Verification items for the finished model (mm, model axes). A direction names the side the tool comes from. Coordinates: 2 decimals unless noted, no trailing zeros. Order: outer loops, then holes, each group sorted by start corner. A loop starts at its lowest first (then second) coordinate and runs counter-clockwise, first axis right, second up. Notation, with made-up numbers: M 4.25,88.25 L 52.25,88.25 A21 ccw 52.25,120.25 Z; hole C -37,34 d9. An arc over 180 degrees is marked long. Use one line per item in the form item = value. Start each with the question number.
```python
from build123d import *

# Parameters (mm, degrees)
BOSS_EXTRUDE1_DEPTH      = 32.1
SKETCH2_R                = 3.075
BOSS_EXTRUDE2_DEPTH      = 1.6
BOSS_EXTRUDE3_START      = 2.1
SKETCH3_R                = 3.075
BOSS_EXTRUDE3_DEPTH      = 2.1
M2_TAPPED_HOLE1_D        = 1.6
M2_TAPPED_HOLE1_DEPTH    = 6
M2_TAPPED_HOLE1_TIP      = 0.480688495
SKETCH6_R                = 1.2
SKETCH6_R_2              = 1.5
BOSS_EXTRUDE4_DEPTH      = 1
SKETCH7_R                = 1
BOSS_EXTRUDE5_DEPTH      = 6
FILLET1_R                = 1
FILLET2_R                = 0.5
BOSS_EXTRUDE6_DEPTH      = 0.15
BOSS_EXTRUDE6_DEPTH_BACK = 0.15
SKETCH9_W                = 1.4
SKETCH9_H                = 1.4
FILLET3_R                = 0.5


with BuildPart() as part:
    # Sketch1 → Boss-Extrude1 (new body)
    with BuildSketch(Plane.XY):
        with BuildLine():
            Line((-6.68954408, 7.7), (6.68954408, 7.7))
            ThreePointArc((6.68954408, 7.7), (10.2, 0), (6.68954408, -7.7))
            Line((6.68954408, -7.7), (-6.68954408, -7.7))
            ThreePointArc((-6.68954408, -7.7), (-10.2, 0), (-6.68954408, 7.7))
        make_face()
    extrude(amount=BOSS_EXTRUDE1_DEPTH)

    # Sketch2 → Boss-Extrude2 (add)
    with BuildSketch(Plane.XY.offset(32.1)):
        Circle(SKETCH2_R)
    extrude(amount=BOSS_EXTRUDE2_DEPTH)

    # Sketch3 → Boss-Extrude3 (add)
    with BuildSketch(Plane(origin=(0, 0, 0), x_dir=(-1, 0, 0), z_dir=(0, 0, -1)).offset(BOSS_EXTRUDE3_START)):
        with Locations(Location((0, 0, 0), (0, 0, 180))):
            Circle(SKETCH3_R)
    extrude(amount=-BOSS_EXTRUDE3_DEPTH)

    # M2 Tapped Hole1
    with Locations(Plane.XY.offset(32.1)):
        with Locations((-6.2, 0), (6.2, 0)):
            Hole(M2_TAPPED_HOLE1_D / 2, depth=M2_TAPPED_HOLE1_DEPTH)
            with Locations((0, 0, -(M2_TAPPED_HOLE1_DEPTH + M2_TAPPED_HOLE1_TIP / 2))):  # 118° drill point
                Cone(0, M2_TAPPED_HOLE1_D / 2, M2_TAPPED_HOLE1_TIP, mode=Mode.SUBTRACT)

    # Sketch6 → Boss-Extrude4 (add)
    with BuildSketch(Plane(origin=(0, 0, 0), x_dir=(-1, 0, 0), z_dir=(0, 0, -1))):
        with Locations(Location((-7.6, 1.69, 0), (0, 0, 180))):
            Circle(SKETCH6_R)
        with Locations(Location((7.6, -1.69, 0), (0, 0, 180))):
            Circle(SKETCH6_R)
        with Locations(Location((-7.6, -1.69, 0), (0, 0, 180))):
            Circle(SKETCH6_R_2)
        with Locations(Location((7.6, 1.69, 0), (0, 0, 180))):
            Circle(SKETCH6_R_2)
    extrude(amount=BOSS_EXTRUDE4_DEPTH)

    # Sketch7 → Boss-Extrude5 (add)
    with BuildSketch(Plane.XY.offset(33.7)):
        Circle(SKETCH7_R)
    extrude(amount=BOSS_EXTRUDE5_DEPTH)

    # Fillet1
    fillet1_edges = [part.edges().sort_by_distance(p)[0] for p in [
        (-10.2, 0, 32.1),
        (0, -7.7, 32.1),
        (10.2, 0, 32.1),
        (0, 7.7, 32.1),
    ]]
    fillet(fillet1_edges, radius=FILLET1_R)

    # Fillet2
    fillet2_edges = [part.edges().sort_by_distance(p)[0] for p in [
        (-3.075, 0, 0),
        (-3.075, 0, -2.1),
    ]]
    fillet(fillet2_edges, radius=FILLET2_R)

    # Sketch9 → Boss-Extrude6 (add, two sides: drawn at the far end of the back side and taken through both)
    # profile 1 of 2: a face of its own
    with BuildSketch(Plane(origin=(0, 0, 0), x_dir=(-0.9761568291371078, 0.2170664527949621, 0), z_dir=(-0.21706645279496206, -0.9761568291371077, 0)).offset(-BOSS_EXTRUDE6_DEPTH_BACK)):
        with BuildLine():
            Line((-8.985634207, 1), (-6.585634207, 1))
            Line((-6.585634207, 1), (-6.585634207, 4.8))
            ThreePointArc((-6.585634207, 4.8), (-6.732080816, 5.153553391), (-7.085634207, 5.3))
            Line((-7.085634207, 5.3), (-8.485634207, 5.3))
            ThreePointArc((-8.485634207, 5.3), (-8.839187597, 5.153553391), (-8.985634207, 4.8))
            Line((-8.985634207, 4.8), (-8.985634207, 1))
        make_face()
        with Locations((-7.785634207, 4.1)):
            Rectangle(SKETCH9_W, SKETCH9_H, mode=Mode.SUBTRACT)
    # profile 2 of 2: a face of its own
    with BuildSketch(Plane(origin=(0, 0, 0), x_dir=(-0.9761568291371078, 0.2170664527949621, 0), z_dir=(-0.21706645279496206, -0.9761568291371077, 0)).offset(-BOSS_EXTRUDE6_DEPTH_BACK)):
        with BuildLine():
            Line((8.985634207, 1), (6.585634207, 1))
            Line((6.585634207, 1), (6.585634207, 4.8))
            ThreePointArc((6.585634207, 4.8), (6.732080816, 5.153553391), (7.085634207, 5.3))
            Line((7.085634207, 5.3), (8.485634207, 5.3))
            ThreePointArc((8.485634207, 5.3), (8.839187597, 5.153553391), (8.985634207, 4.8))
            Line((8.985634207, 4.8), (8.985634207, 1))
        make_face()
        with Locations((7.785634207, 4.1)):
            Rectangle(SKETCH9_W, SKETCH9_H, mode=Mode.SUBTRACT)
    extrude(amount=BOSS_EXTRUDE6_DEPTH + BOSS_EXTRUDE6_DEPTH_BACK)

    # Fillet3
    fillet3_edges = [part.edges().sort_by_distance(p)[0] for p in [
        (-6.91669022, 1.538053483, -4.8),
        (8.28330978, -1.841946517, -4.8),
        (6.91669022, -1.538053483, -4.8),
        (6.91669022, -1.538053483, -3.4),
        (8.28330978, -1.841946517, -3.4),
        (-8.28330978, 1.841946517, -4.8),
        (-8.28330978, 1.841946517, -3.4),
        (-6.91669022, 1.538053483, -3.4),
    ]]
    fillet(fillet3_edges, radius=FILLET3_R)


solid = part.part
```
1. Release check for a two-part mould opening along X. For faces 1 (the cylindrical face through (-10.2, -0.1, 15.3)), 2 (the cylindrical face through (7, 0, 29)), 3 (the flat face through (7.649, -1.547, -3.18)) record: pulls with the +X half, pulls with the -X half, needs draft (parallel to the pull), parting line crosses it, or undercut.
2. Depth check by flat-ended pin: P1, Ø1.2, axis at x = 7.5, y = 1.5, coming from the -Z side; P2, Ø1, axis at x = 6.2, y = 0, coming from the +Z side; P3, Ø2, axis at y = -4, z = 24.5, coming from the -X side. Enter the tip coordinate at first touch or a pass-through.
3. Tool access check on faces 4 (the flat face through (-7.649, 1.547, -3.18)), 5 (the flat face through (8, 2, -1)), 6 (the flat face through (7.58, -1.84, -3.18)), 7 (the flat face through (8, -1, -1)), 8 (the flat face through (-1, 1, 33.7)). Record the directions out of +Z, -Z, +X, -X, +Y, -Y that give a thin tool (end or side, any length) a straight path to the whole face; none if there is none.
4. Cross-section at C-C on z = 18. Enter the section's corners in (x, y), and give its area (3 significant figures).
5. Cross-section at A-A on z = 28. Enter the section's corners in (x, y), and give its area (3 significant figures).
6. Cross-section at B-B on x = 0. Enter the section's corners in (y, z) (3 decimals), and give its area (3 significant figures).
7. Cross-section at D-D on z = 37.5. Enter the section's corners in (x, y).
8. Material ranges on line 1 along Y through (x, z) = (-6.2, 30.65); line 2 along Z through (x, y) = (-1.5, 1.5); line 3 along Z through (x, y) = (9.25, 1.25), recorded low to high.
Final values:
q1.face_1 = pulls with the -X half
q1.face_2 = undercut
q1.face_3 = pulls with the +X half
q2.P1 = -1
q2.P2 = 25.92
q2.P3 = -9.75
q3.face_4 = -Z, -X, -Y
q3.face_5 = -Z, +X, +Y
q3.face_6 = -Z, -Y
q3.face_7 = -Z
q3.face_8 = +Z
q4.outline = M -6.69,-7.7 L 6.69,-7.7 A10.2 ccw 6.69,7.7 L -6.69,7.7 A10.2 ccw Z
q4.area = 281 mm2
q5.outline = M -6.69,-7.7 L 6.69,-7.7 A10.2 ccw 6.69,7.7 L -6.69,7.7 A10.2 ccw Z; hole C -6.2,0 d1.6; hole C 6.2,0 d1.6
q5.area = 277 mm2
q6.outline = M -7.7,0 L -3.575,0 A0.5 cw -3.075,-0.5 L -3.075,-1.6 A0.5 ccw -2.575,-2.1 L 2.575,-2.1 A0.5 ccw 3.075,-1.6 L 3.075,-0.5 A0.5 cw 3.575,0 L 7.7,0 L 7.7,31.1 A1 ccw 6.7,32.1 L 3.075,32.1 L 3.075,33.7 L 1,33.7 L 1,39.7 L -1,39.7 L -1,33.7 L -3.075,33.7 L -3.075,32.1 L -6.7,32.1 A1 ccw -7.7,31.1 Z
q6.area = 529 mm2
q7.outline = C 0,0 d2
q8.line_1 = -7.7 to -0.8, 0.8 to 7.7
q8.line_2 = -2.1 to 33.7
q8.line_3 = 0 to 32.09
